Here's the drawing with two shaded views (mm, measured from the low corner). I have some questions. A direction names the side the tool comes from. Round coordinates to 2 decimals unless told otherwise and drop trailing zeros. Loops run counter-clockwise (first coordinate to the right, second up) from the corner with the lowest first, then second, coordinate; pieces in that order, holes last. Notation, with made-up numbers: M 56.5,-8.75 L 109.5,-8.75 A25 cw 109.5,6.25 Z; hole C 88.25,-8 d2. An arc over 180 degrees is marked long. Answer as CSV lines item,"result".
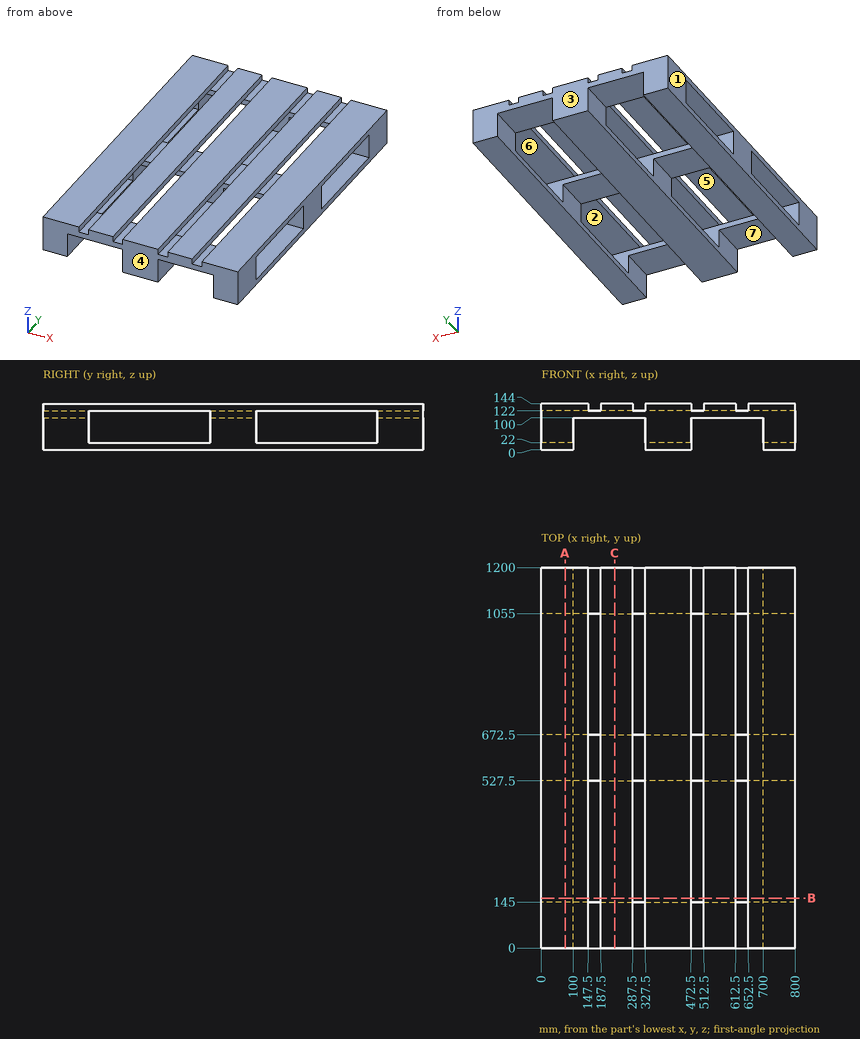
1. Which directions (+Z, -Z, +X, -X, +Y, -Y) give clear straight access to the entire face, cutting with the end or side of a thin tool? Please do the marked faces 5, 6 and 7.
Evaluation:
face 5,"-Z, +X, -X"
face 6,"+X, -X"
face 7,"-Z, +Y, -Y"
2. For P1, Ø12, axis at x = 171.5, y = 599.5, coming from the +Z side, with a flat end and sliding along its axis, tell me the tip position at first contact or that it passes through.
Evaluation:
P1,"stops at z = 122"
3. I want a section at C-C, the plane x = 231. Please give me the cut outline in (y, z), and give its area (3 significant figures).
Evaluation:
outline,"M 0,100 L 145,100 L 145,122 L 527.5,122 L 527.5,100 L 672.5,100 L 672.5,122 L 1055,122 L 1055,100 L 1200,100 L 1200,144 L 0,144 Z"
area,"36,000 mm²"
4. If I drill on line 1 (Y direction, x = 764, z = 69.5); line 2 (X direction, y = 125, z = 66.5); line 3 (X direction, y = 1039.5, z = 123), over which ranges is the centre line in solid material (lowest first)? Write a range as [from, to].
Evaluation:
line 1,"y = [0, 145], [527.5, 672.5], [1055, 1200]"
line 2,"x = [0, 100], [327.5, 472.5], [700, 800]"
line 3,"x = [0, 147.5], [187.5, 287.5], [327.5, 472.5], [512.5, 612.5], [652.5, 800]"
5. I want a section at A-A, the plane x = 75. Please give me the cut outline in (y, z).
Evaluation:
outline,"M 0,0 L 1200,0 L 1200,144 L 0,144 Z; hole M 145,22 L 527.5,22 L 527.5,122 L 145,122 Z; hole M 672.5,22 L 1055,22 L 1055,122 L 672.5,122 Z"
6. I want a section at B-B, the plane y = 157.5. Count the separate pieces of the cut face and the enclosed holes in it, and give its area (3 significant figures).
Evaluation:
separate pieces,"8"
enclosed holes,"0"
area,"21,700 mm²"
7. We'd pull the mould along Y, two halves only. Please class the marked faces 1, 2, 3 and 4: pulls with the +Y half, pulls with the -Y half, needs draft (parallel to the pull), parting line crosses it, or undercut.
Evaluation:
face 1,"needs draft"
face 2,"undercut"
face 3,"pulls with the +Y half"
face 4,"pulls with the -Y half"
